Read the model definition and answer for the solid it produces. Units are mm, in the model's axes. Face numbers are marked on the shaded views. A direction names the side the tool comes from. Give positions to 0.01 mm unless a question says otherwise; leave off trailing zeros. Loops run counter-clockwise (first coordinate to the right, second up) from the corner with the lowest first, then second, coordinate; pieces in that order, holes last. Notation, with made-up numbers: (46, -31) -> (50, -31) arc R17 ccw to (50, -23) -> close; hole circle Ø4 at (34, 66). An arc over 180 degrees is marked (long way). Write each question's results on one line, items separated by ' | '. Start each with the question number.
Item 1: Section B-B on y = 14.5 is taken. Write down the section's boundary in (x, z).
Item 2: Section A-A on y = 2 is taken. Write down the section's boundary in (x, z).
Item 3: Section D-D on z = -4.25 is taken. Write down the section's boundary in (x, y), and give its area (3 significant figures).
Item 4: Section C-C on x = -7.5 is taken. Write down the section's boundary in (y, z), and give its area (3 significant figures).
Item 5: Which of the six approach directions +Z, -Z, +X, -X, +Y, -Y give full straight-line access (tool end or side, diameter ignored) to the marked faces 1, 2 and 3?
Item 6: Find the intervals of material crossed by line 1 (Y direction, x = 1, z = 3.5); line 2 (Y direction, x = -0.25, z = 0); line 3 (X direction, y = -7.25, z = 0), in increasing order.
Item 7: Each of these flat-tipped pins is pushed along its axis until it touches: P1, Ø5, axis at x = 1.5, z = 1.5, coming from the +Y side; P2, Ø6.5, axis at x = -0.5, z = -1.5, coming from the -Y side; P3, Ø2, axis at x = -6.5, y = 24.5, coming from the +Z side; P4, Ø2, axis at y = 0, z = -1.5, coming from the -X side. Where does it stop, or does it pass through?
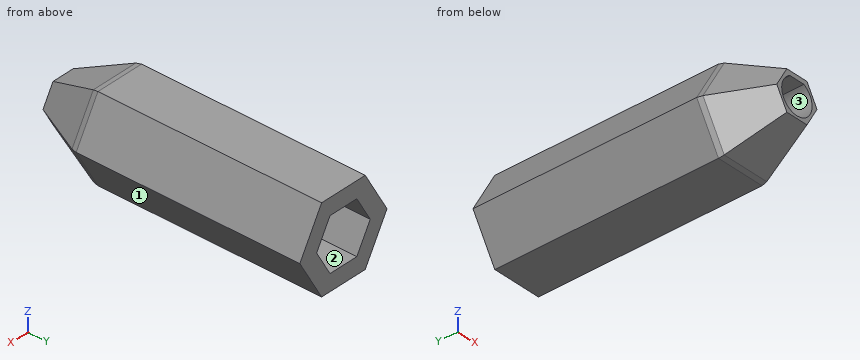
Autodesk Inventor part; units mm, degrees
ref_plane "YZ Plane" through (0, 0, 0) normal (1, 0, 0) x (0, 1, 0)
ref_plane "XZ Plane" through (0, 0, 0) normal (0, 1, 0) x (-1, 0, 0)
ref_plane "XY Plane" through (0, 0, 0) normal (0, 0, 1) x (1, 0, 0)
sketch "Boceto11" plane through (0, 0, 0) normal (0, 1, 0) x (-1, 0, 0)
  line L0 (0, 0) -> (5.6, 0)
  line L1 (5.6, 0) -> (2.8, -4.8497)
  line L2 (2.8, -4.8497) -> (-2.8, -4.8497)
  line L3 (-2.8, -4.8497) -> (-5.6, 0)
  line L4 (-5.6, 0) -> (-2.8, 4.8497)
  line L5 (-2.8, 4.8497) -> (2.8, 4.8497)
  line L6 (2.8, 4.8497) -> (5.6, 0)
  line L7 (5.6, 0) -> (9.1, 0)
  line L8 (9.1, 0) -> (4.55, -7.8808)
  line L9 (4.55, -7.8808) -> (-4.55, -7.8808)
  line L10 (-4.55, -7.8808) -> (-9.1, 0)
  line L11 (-9.1, 0) -> (-4.55, 7.8808)
  line L12 (-4.55, 7.8808) -> (4.55, 7.8808)
  line L13 (4.55, 7.8808) -> (9.1, 0)
  dimension "d42" = 5.6
  dimension "d43" = 3.5
extrude "Extrusión10" add sketch "Boceto11" along normal blind 32
sketch "Boceto16" plane through (0, 0, 0) normal (0, -1, 0) x (1, 0, 0)
  line L0 (4.55, 7.8808) -> (9.1, 0)
  line L1 (9.1, 0) -> (4.55, -7.8808)
  line L2 (4.55, -7.8808) -> (-4.55, -7.8808)
  line L3 (-4.55, -7.8808) -> (-9.1, 0)
  line L4 (-9.1, 0) -> (-4.55, 7.8808)
  line L5 (-4.55, 7.8808) -> (4.55, 7.8808)
  line L6 (4.55, 7.8808) -> (9.1, 0)
  point P0 (0, 0)
  point P1 (0, 0)
extrude "Extrusión14" add sketch "Boceto16" along normal blind 10 draft -23
sketch "Boceto19" plane through (0, -10, 0) normal (0, -1, 0) x (1, 0, 0)
  line L0 (-2.0993, 3.6361) -> (2.0993, 3.6361)
  line L1 (2.0993, -3.6361) -> (-2.0993, -3.6361)
  line L2 (2.0993, 3.6361) -> (4.1986, 0)
  line L3 (-4.55, -7.8808) -> (-2.0993, -3.6361)
  line L4 (-4.1986, 0) -> (-2.0993, 3.6361)
  arc A0 (-1.4491, 2.825) -> (1.4491, 2.825) centre (0, 0) ccw
  line L5 (0, 2.825) -> (-1.4491, 2.825)
  line L6 (0, 2.825) -> (1.4491, 2.825)
extrude "Extrusión16" cut sketch "Boceto19" against normal blind 15
sketch "Boceto20" plane through (0, 0, 0) normal (0, 1, 0) x (1, 0, 0)
  line L0 (-4.55, -7.8808) -> (-2.0993, -3.6361)
  line L1 (-2.7798, -4.8148) -> (-5.5597, 0)
  line L2 (-5.5597, 0) -> (-2.7798, 4.8148)
  line L3 (-2.7798, 4.8148) -> (2.7798, 4.8148)
  line L4 (2.7798, 4.8148) -> (5.5597, 0)
  line L5 (5.5597, 0) -> (2.7798, -4.8148)
  line L6 (2.7798, -4.8148) -> (-2.7798, -4.8148)
  point P0 (0, 0)
  point P1 (0, 0)
extrude "Extrusión17" add sketch "Boceto20" along normal blind 5
sketch "Boceto21" plane through (0, 32, 0) normal (0, 1, 0) x (1, 0, 0)
  line L0 (-5.6, 0) -> (-2.8, 4.8497)
  line L1 (-2.8, 4.8497) -> (2.8, 4.8497)
  line L2 (2.8, 4.8497) -> (5.6, 0)
  line L3 (5.6, 0) -> (2.8, -4.8497)
  line L4 (2.8, -4.8497) -> (-2.8, -4.8497)
  line L5 (-2.8, -4.8497) -> (-5.6, 0)
  line L6 (-2.8, -4.8497) -> (-5.6, 0)
  line L7 (-9.1, 0) -> (-4.55, -7.8808)
  line L8 (-4.55, -7.8808) -> (-9.1, 0)
  line L9 (-4.55, 7.8808) -> (-9.1, 0)
  line L10 (-9.1, 0) -> (-4.55, 7.8808)
  line L11 (4.55, 7.8808) -> (2.0993, 3.6361)
  line L12 (-4.55, 7.8808) -> (4.55, 7.8808)
  line L13 (4.55, -7.8808) -> (9.1, 0)
  line L14 (4.55, 7.8808) -> (9.1, 0)
  line L15 (9.1, 0) -> (4.55, -7.8808)
  line L16 (4.55, -7.8808) -> (-4.55, -7.8808)
  point P0 (0, 0)
  point P1 (0, 0)
  point P2 (0, 0)
chamfer "Chaflán1" distance 0.5 angle 45 6 edges at (0, 0, -7.8808) (-6.825, 0, -3.9404) (6.825, 0, -3.9404) (-6.825, 0, 3.9404) (0, 0, 7.8808) (6.825, 0, 3.9404)
extrude "Extrusión19" add sketch "Boceto21" along normal blind 10
properties part number "Bobinatge - acoplament eix"
Findings:
1) outline: (-9.1, 0) -> (-4.55, -7.88) -> (4.55, -7.88) -> (9.1, 0) -> (4.55, 7.88) -> (-4.55, 7.88) -> close; hole (-5.6, 0) -> (-2.8, -4.85) -> (2.8, -4.85) -> (5.6, 0) -> (2.8, 4.85) -> (-2.8, 4.85) -> close
2) outline: (-9.1, 0) -> (-4.55, -7.88) -> (4.55, -7.88) -> (9.1, 0) -> (4.55, 7.88) -> (-4.55, 7.88) -> close; (-5.56, 0) -> (-2.78, -4.81) -> (2.78, -4.81) -> (5.56, 0) -> (2.78, 4.81) -> (-2.78, 4.81) -> close; hole (-5.6, 0) -> (-2.8, -4.85) -> (2.8, -4.85) -> (5.6, 0) -> (2.8, 4.85) -> (-2.8, 4.85) -> close
3) outline: (-6.65, 0.5) -> (-6.42, -0.46) -> (-2.45, -8.55) -> (2.45, -8.55) -> (6.42, -0.46) -> (6.65, 0.5) -> (6.65, 42) -> (3.15, 42) -> (3.15, 0) -> (3.11, 0) -> (3.11, 5) -> (-3.11, 5) -> (-3.11, 0) -> (-3.15, 0) -> (-3.15, 42) -> (-6.65, 42) -> close | area: 403 mm2
4) outline: (-3.26, 0) -> (-0.46, -2.38) -> (0.5, -2.77) -> (42, -2.77) -> (42, 2.77) -> (0.5, 2.77) -> (-0.46, 2.38) -> close | area: 242 mm2
5) face 1: -Z, +X, +Y, -Y | face 2: +Y | face 3: -Y
6) line 1: -10 to 5 | line 2: 0 to 5 | line 3: -5.55 to -3.17, 3.17 to 5.55
7) P1: y = 5 | P2: y = -10 | P3: z = 6.24 | P4: x = -8.74
